from build123d import *

# Parameters (mm, degrees)
EXTRUDE_1_DEPTH     = 3
SKETCH_2_W          = 16
SKETCH_2_H          = 5
EXTRUDE_2_DEPTH     = 51
EXTRUDE_START       = 3
EXTRUDE_3_DEPTH     = 3
FILLET_1_R          = 1
CHAMFER_1_SIZE      = 0.5
SKETCH_4_W          = 8
SKETCH_4_H          = 38
CUT_EXTRUDE_1_DEPTH = 55.817880295
FILLET_2_R          = 3


with BuildPart() as part:
    # 草图1 → 凸台-拉伸1 (new body)
    with BuildSketch(Plane.XY):
        with BuildLine():
            Line((-4, 1.5), (4, 1.5))
            ThreePointArc((4, 1.5), (5.5, 0), (4, -1.5))
            Line((4, -1.5), (-4, -1.5))
            ThreePointArc((-4, -1.5), (-5.5, 0), (-4, 1.5))
        make_face()
    extrude(amount=EXTRUDE_1_DEPTH)

    # 草图2 → 凸台-拉伸2 (add)
    with BuildSketch(Plane(origin=(0, 0, 0), x_dir=(-1, 0, 0), z_dir=(0, 0, -1))):
        with Locations((0, 1)):
            Rectangle(SKETCH_2_W, SKETCH_2_H)
    extrude(amount=EXTRUDE_2_DEPTH)

    # 草图3 → 凸台-拉伸3 (add)
    with BuildSketch(Plane(origin=(0, 0, -51), x_dir=(-1, 0, 0), z_dir=(0, 0, -1)).offset(EXTRUDE_START)):
        with BuildLine():
            Line((-4, 1.5), (4, 1.5))
            ThreePointArc((4, 1.5), (5.5, 0), (4, -1.5))
            Line((4, -1.5), (-4, -1.5))
            ThreePointArc((-4, -1.5), (-5.5, 0), (-4, 1.5))
        make_face()
    extrude(amount=-EXTRUDE_3_DEPTH)

    # 圆角1
    fillet_1_edges = [part.edges().sort_by_distance(p)[0] for p in [
        (-8, -1.5, -25.5),
        (-8, 3.5, -25.5),
        (8, 3.5, -25.5),
        (8, -1.5, -25.5),
    ]]
    fillet(fillet_1_edges, radius=FILLET_1_R)

    # 倒角1
    chamfer_1_edges = [part.edges().sort_by_distance(p)[0] for p in [
        (5.5, 0, 3),
        (0, 1.5, 3),
        (5.5, 0, -54),
        (0, -1.5, -54),
        (-5.5, 0, -54),
        (0, 1.5, -54),
        (-5.5, 0, 3),
        (0, -1.5, 3),
    ]]
    chamfer(chamfer_1_edges, length=CHAMFER_1_SIZE)

    # 草图4 → 切除-拉伸1 (cut, through all)
    with BuildSketch(Plane.XZ.offset(1.5)):
        with Locations((0, -25)):
            Rectangle(SKETCH_4_W, SKETCH_4_H)
    extrude(amount=-CUT_EXTRUDE_1_DEPTH, mode=Mode.SUBTRACT)

    # 圆角2
    fillet_2_edges = [part.edges().sort_by_distance(p)[0] for p in [
        (4, 1, -6),
        (4, 1, -44),
        (-4, 1, -44),
        (-4, 1, -6),
    ]]
    fillet(fillet_2_edges, radius=FILLET_2_R)


solid = part.part
Source: CAD feature listing. Evaluate the final solid. Frame: model axes, mm. A direction names the side the tool comes from. Round coordinates to 2 decimals unless told otherwise and drop trailing zeros. Write each loop counter-clockwise with the first axis right and the second up, starting at its lowest first coordinate (ties: lowest second). Pieces come first, ordered by that corner, then holes. Notation, with made-up numbers: (-25, 58.5) - (1, 58.5) arc R24 cw to (1, 69.5) - close; hole circle Ø6 at (-4, 88.5). An arc over 180 degrees is marked (long way). Use CSV: the item, a comma, the result in double quotes. Start each with the question number.
(1) Material intervals for probe 1 along X at (y, z) = (0.95, -18); probe 2 along Z at (x, y) = (-0.5, 0.9); probe 3 along Z at (x, y) = (6.5, 1.05), sorted ascending. Write a range as [from, to].
(2) First-contact query: pin 1 Ø1.6 at (x, y) = (-0.5, 2) entering from +Z; pin 2 Ø1.2 at (x, z) = (-1, 1) entering from +Y; pin 3 Ø1.6 at (x, y) = (0, 2) entering from -Z. Flat tips, straight axial feed; report the tip coordinate or a pass-through.
(3) Cut plane D-D, the plane y = 3. Return loops of the section in (x, z).
(4) Cut plane C-C, the plane y = 0. Return loops of the section in (x, z).
(5) Cut plane A-A, the plane x = 0. Return loops of the section in (y, z), and give its area (3 significant figures).
(6) Set-up query: faces 1 (the face through (5.5, 0, -52.3)), 2 (the face through (-5.5, 0, -52.3)), 3 (the face through (-3.14, 1.04, -6.9)). Return all of +Z, -Z, +X, -X, +Y, -Y with unobstructed straight access to the full face (end or side cutting, diameter ignored); none if empty.
(7) Cut plane B-B, the plane z = -22. Return loops of the section in (x, y), and give its area (3 significant figures).
(8) Mould query, pull axis X, two halves, no side actions, for faces 4 (the face through (-3.14, 1.04, -43.1)), 5 (the face through (0, 0, 3)), 6 (the face through (-5.5, 0, 1.2)), 7 (the face through (5.14, 0.02, 2.86)). Classes: pulls with the +X half, pulls with the -X half, needs draft (parallel to the pull), parting line crosses it, or undercut.
Geometry says:
1,probe 1,"[-8, -4], [4, 8]"
1,probe 2,"[-54, -44], [-6, 3]"
1,probe 3,"[-51, 0]"
2,pin 1,"z = 2.8"
2,pin 2,"y = 1.5"
2,pin 3,"z = -53.8"
3,outline,"(-7.87, -51) - (7.87, -51) - (7.87, 0) - (-7.87, 0) - close; hole (-4, -41) arc R3 ccw to (-1, -44) - (1, -44) arc R3 ccw to (4, -41) - (4, -9) arc R3 ccw to (1, -6) - (-1, -6) arc R3 ccw to (-4, -9) - close"
4,outline,"(-8, -51) - (-5.5, -51) - (-5.5, -53.5) - (-5, -54) - (5, -54) - (5.5, -53.5) - (5.5, -51) - (8, -51) - (8, 0) - (5.5, 0) - (5.5, 2.5) - (5, 3) - (-5, 3) - (-5.5, 2.5) - (-5.5, 0) - (-8, 0) - close; hole (-4, -41) arc R3 ccw to (-1, -44) - (1, -44) arc R3 ccw to (4, -41) - (4, -9) arc R3 ccw to (1, -6) - (-1, -6) arc R3 ccw to (-4, -9) - close"
5,outline,"(-1.5, -53.5) - (-1, -54) - (1, -54) - (1.5, -53.5) - (1.5, -51) - (3.5, -51) - (3.5, -44) - (-1.5, -44) - close; (-1.5, -6) - (3.5, -6) - (3.5, 0) - (1.5, 0) - (1.5, 2.5) - (1, 3) - (-1, 3) - (-1.5, 2.5) - close"
5,area,"82.5 mm²"
6,face 1,"-Z, +X"
6,face 2,"-Z, -X"
6,face 3,"+Y, -Y"
7,outline,"(-8, -0.5) arc R1 ccw to (-7, -1.5) - (-4, -1.5) - (-4, 3.5) - (-7, 3.5) arc R1 ccw to (-8, 2.5) - close; (4, -1.5) - (7, -1.5) arc R1 ccw to (8, -0.5) - (8, 2.5) arc R1 ccw to (7, 3.5) - (4, 3.5) - close"
7,area,"39.1 mm²"
8,face 4,"undercut"
8,face 5,"needs draft"
8,face 6,"pulls with the -X half"
8,face 7,"pulls with the +X half"
